Answer from the drawing. Dimensions are ordinates in mm from the lowest x, y and z of the part. Coordinates: 2 decimals unless noted, no trailing zeros. Write each loop counter-clockwise with the first axis right and the second up, starting at its lowest first coordinate (ties: lowest second). Pieces come first, ordered by that corner, then holes. Notation, with made-up numbers: (89.25, 54.5) - (142.25, 54.5) arc R21 cw to (142.25, 66.5) - close; hole circle Ø9 at (11, 60). An arc over 180 degrees is marked (long way). Use a Markdown table: item, result.
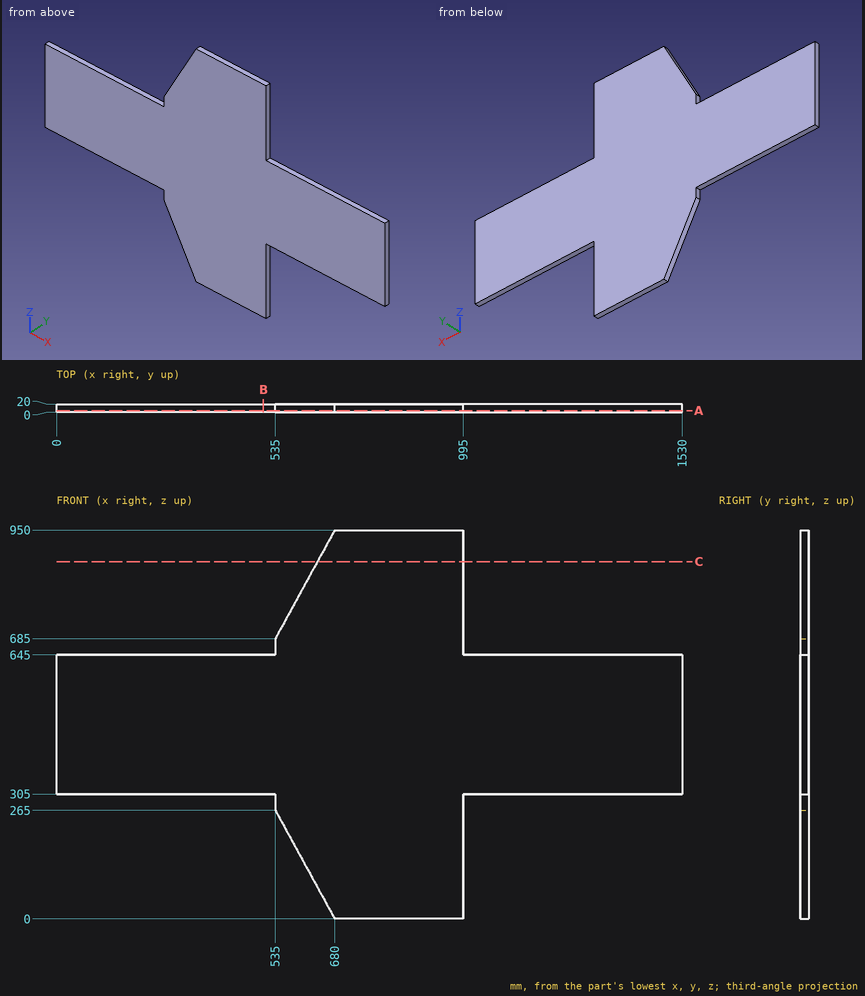
(1) A cutting plane is placed at C-C, the plane z = 873. Write down the section's boundary in (x, y), and give its area (3 significant figures).
Report:
| item | result |
|---|---|
| outline | (637.87, 0) - (995, 0) - (995, 20) - (637.87, 20) - close |
| area | 7,140 mm² |
(2) A cutting plane is placed at B-B, the plane x = 506. Write down the section's boundary in (y, z).
Report:
| item | result |
|---|---|
| outline | (0, 305) - (20, 305) - (20, 645) - (0, 645) - close |
(3) Straight lines are drawn through the part: L1, parallel to Z at x = 1301, y = 2.5; L2, parallel to X at y = 7.5, z = 114; L3, parallel to X at y = 16.5, z = 68. For each, find the intervals that lie inside material, in ascending order.
Report:
| item | result |
|---|---|
| L1 | z = 305 to 645 |
| L2 | x = 617.62 to 995 |
| L3 | x = 642.79 to 995 |
(4) Each of these flat-tipped pins is pushed along its axis until it touches: P1, Ø12, axis at y = 14, z = 157, coming from the +X side; P2, Ø12, axis at x = 1376.5, y = 10.5, coming from the +Z side; P3, Ø1.5, axis at y = 10, z = 792, coming from the -X side. Where does it stop, or does it pass through?
Report:
| item | result |
|---|---|
| P1 | stops at x = 995 |
| P2 | stops at z = 645 |
| P3 | stops at x = 593.14 |
(5) A cutting plane is placed at A-A, the plane y = 3.5. Write down the section's boundary in (x, z), and give its area (3 significant figures).
Report:
| item | result |
|---|---|
| outline | (0, 305) - (535, 305) - (535, 265) - (680, 0) - (995, 0) - (995, 305) - (1530, 305) - (1530, 645) - (995, 645) - (995, 950) - (680, 950) - (535, 685) - (535, 645) - (0, 645) - close |
| area | 762,000 mm² |
